Read the model definition and answer for the solid it produces. Units are mm, in the model's axes. A direction names the side the tool comes from. Round coordinates to 2 decimals unless told otherwise and drop trailing zeros. Write each loop counter-clockwise with the first axis right and the second up, starting at its lowest first coordinate (ties: lowest second). Pieces come first, ordered by that corner, then holes. Notation, with made-up numbers: (-12, 88.25) -> (47, 88.25) arc R18 ccw to (47, 102.25) -> close; hole circle Ø1 at (58.5, 14.25). An arc over 180 degrees is marked (long way). Return JSON: item names as keys, results as strings.
from build123d import *

# Parameters (mm, degrees)
F0_W     = 181
F0_H     = 94.5
F1_DEPTH = 46
F2_R     = 27
F3_T     = -2
F4_R     = 12
F5_DEPTH = 105


with BuildPart() as f1:
    # F0 (on Top) → F1 (new body)
    with BuildSketch(Plane.XY):
        with Locations((-9.7413412556, -21.9173085093)):
            Rectangle(F0_W, F0_H)
    extrude(amount=-F1_DEPTH)

    # F2
    f2_edges = [f1.edges().sort_by_distance(p)[0] for p in [
        (80.758659, 25.332691, -23),
        (-100.241341, 25.332691, -23),
        (-100.241341, -69.167309, -23),
        (80.758659, -69.167309, -23),
    ]]
    fillet(f2_edges, radius=F2_R)

    # F3
    f3_openings = [f1.faces().sort_by_distance(p)[0] for p in [
        (-9.741341, -21.917309, 0),
    ]]
    offset(amount=F3_T, openings=f3_openings)

    # F4 (on face) → F5 (cut)
    with BuildSketch(Plane.XZ.offset(69.1673085093)):
        with Locations((-9.7413412556, 0)):
            Circle(F4_R)
    extrude(amount=-F5_DEPTH, mode=Mode.SUBTRACT)


solid = f1.part
Item 1: Section D-D (x = 36.5) is taken. Give the vertices of the cut face in (y, z).
Worked answers:
{"outline": "(-69.17, -46) -> (25.33, -46) -> (25.33, 0) -> (23.33, 0) -> (23.33, -44) -> (-67.17, -44) -> (-67.17, 0) -> (-69.17, 0) -> close"}
Item 2: Section B-B (y = -39.5) is taken. Give the vertices of the cut face in (x, z), then the cut area to 3 significant figures.
Worked answers:
{"outline": "(-100.24, -46) -> (80.76, -46) -> (80.76, 0) -> (78.76, 0) -> (78.76, -44) -> (-98.24, -44) -> (-98.24, 0) -> (-100.24, 0) -> close", "area": "538 mm2"}
Item 3: For a pull along X with two mould halves and no side action, classify faces 1 (the flat face through (-11, -21, -44)), 2 (the flat face through (-11, 25.333, -23)), 3 (the cylindrical face through (-92.542, 17.213, -23.322)) as released by +X, released by -X, zero draft, split by the parting line, or undercut.
Worked answers:
{"face 1": "undercut", "face 2": "zero draft", "face 3": "released by -X"}
Item 4: Straight lines are drawn through the part: L1, parallel to Y at x = 45, z = -8; L2, parallel to X at y = -14.5, z = -19.5; L3, parallel to Z at x = -67, y = -57. For each, find the intervals that lie inside material, in ascending order. Write a range as [from, to].
Worked answers:
{"L1": "y = [-69.17, -67.17], [23.33, 25.33]", "L2": "x = [-100.24, -98.24], [78.76, 80.76]", "L3": "z = [-46, -44]"}
Item 5: Section C-C (z = -8) is taken. Give the vertices of the cut face in (x, y).
Worked answers:
{"outline": "(-100.24, -42.17) arc R27 ccw to (-73.24, -69.17) -> (-18.69, -69.17) -> (-18.69, -67.17) -> (-73.24, -67.17) arc R25 cw to (-98.24, -42.17) -> (-98.24, -1.67) arc R25 cw to (-73.24, 23.33) -> (-18.69, 23.33) -> (-18.69, 25.33) -> (-73.24, 25.33) arc R27 ccw to (-100.24, -1.67) -> close; (-0.8, -69.17) -> (53.76, -69.17) arc R27 ccw to (80.76, -42.17) -> (80.76, -1.67) arc R27 ccw to (53.76, 25.33) -> (-0.8, 25.33) -> (-0.8, 23.33) -> (53.76, 23.33) arc R25 cw to (78.76, -1.67) -> (78.76, -42.17) arc R25 cw to (53.76, -67.17) -> (-0.8, -67.17) -> close"}
Item 6: A tool of negligible diameter and unlimited length cuts with its end or side. For faces 4 (the cylindrical face through (71.63, 15.815, -22.308)), 5 (the flat face through (-11, -69.167, -23)), from which of +Z, -Z, +X, -X, +Y, -Y can it reach the whole face along a straight path? Write none if from no direction.
Worked answers:
{"face 4": "+Z", "face 5": "+Z, -Z, +X, -X, -Y"}
Item 7: Flat-ended cylindrical pins translate along their axes: pin 1 (2 mm diameter, centred on x = -52, y = -22.5, fed in from +Z); pin 2 (6 mm diameter, centred on x = -79.5, z = -27.5, fed in from -Y); pin 3 (8 mm diameter, centred on y = 6.5, z = -9.5, fed in from -X). Find the tip coordinate at first contact, or state that the pin passes through.
Worked answers:
{"pin 1": "stops at z = -44", "pin 2": "stops at y = -68.97", "pin 3": "stops at x = -99.92"}
Item 8: Section A-A (z = -26) is taken. Give the vertices of the cut face in (x, y).
Worked answers:
{"outline": "(-100.24, -42.17) arc R27 ccw to (-73.24, -69.17) -> (53.76, -69.17) arc R27 ccw to (80.76, -42.17) -> (80.76, -1.67) arc R27 ccw to (53.76, 25.33) -> (-73.24, 25.33) arc R27 ccw to (-100.24, -1.67) -> close; hole (-98.24, -42.17) arc R25 ccw to (-73.24, -67.17) -> (53.76, -67.17) arc R25 ccw to (78.76, -42.17) -> (78.76, -1.67) arc R25 ccw to (53.76, 23.33) -> (-73.24, 23.33) arc R25 ccw to (-98.24, -1.67) -> close"}
